Read the model definition and answer for the solid it produces. Units are mm, in the model's axes. A direction names the side the tool comes from. Coordinates: 2 decimals unless noted, no trailing zeros. Loops run counter-clockwise (first coordinate to the right, second up) from the corner with the lowest first, then second, coordinate; pieces in that order, holes last.
from build123d import *

# Parameters (mm, degrees)
F1_DEPTH = 7.5
F2_W     = 25
F2_H     = 2
F2_W_2   = 87.9392416629
F3_DEPTH = 127.501
F4_DEPTH = 7.5
F5_D     = 3
F5_DEPTH = 13.5
F5_TIP   = 0.9012909285
F7_R     = 2.6
F8_DEPTH = 15
F6_R     = 2.55
F9_DEPTH = 12.5


with BuildPart() as f1:
    # F0 (on Front) → F1 (new body, symmetric)
    with BuildSketch(Plane.XZ):
        with BuildLine():
            ThreePointArc((0, 127.5), (5.3033008589, 125.3033008589), (7.5, 120))
            ThreePointArc((7.5, 120), (5.3033008589, 114.6966991411), (0, 112.5))
            Line((0, 112.5), (108.7850481272, 112.5))
            Line((108.7850481272, 112.5), (108.7850481272, 127.5))
            Line((108.7850481272, 127.5), (0, 127.5))
        make_face()
        with BuildLine():
            Line((120, 127.5), (108.7850481272, 127.5))
            Line((108.7850481272, 127.5), (108.7850481272, 112.5))
            Line((108.7850481272, 112.5), (120, 112.5))
            ThreePointArc((120, 112.5), (127.5, 120), (120, 127.5))
        make_face()
        with BuildLine():
            ThreePointArc((0, 112.5), (5.3033008589, 114.6966991411), (7.5, 120))
            ThreePointArc((7.5, 120), (5.3033008589, 125.3033008589), (0, 127.5))
            ThreePointArc((0, 127.5), (-7.5, 120), (0, 112.5))
        make_face()
        with BuildLine():
            Line((162.6379891518, 127.5), (120, 127.5))
            ThreePointArc((120, 127.5), (127.5, 120), (120, 112.5))
            Line((120, 112.5), (124.3643918131, 112.5))
            ThreePointArc((124.3643918131, 112.5), (126.7854456219, 110.6232964421), (125.5716191931, 107.8107987637))
            Line((125.5716191931, 107.8107987637), (-3.6216821402, 36.5676037088))
            ThreePointArc((-3.6216821402, 36.5676037088), (3.813619275, 36.4580421202), (7.5, 30))
            ThreePointArc((7.5, 30), (6.4580421202, 26.186380725), (3.6216821402, 23.4323962912))
            Line((3.6216821402, 23.4323962912), (163.8452165318, 111.7871050513))
            ThreePointArc((163.8452165318, 111.7871050513), (164.7906698585, 112.7050998626), (165.1379891518, 113.9763062876))
            Line((165.1379891518, 113.9763062876), (165.1379891518, 125))
            ThreePointArc((165.1379891518, 125), (164.4057561047, 126.767766953), (162.6379891518, 127.5))
        make_face()
        with BuildLine():
            ThreePointArc((7.5, 30), (3.813619275, 36.4580421202), (-3.6216821402, 36.5676037088))
            ThreePointArc((-3.6216821402, 36.5676037088), (-6.5676037088, 26.3783178598), (3.6216821402, 23.4323962912))
            ThreePointArc((3.6216821402, 23.4323962912), (6.4580421202, 26.186380725), (7.5, 30))
        make_face()
    extrude(amount=F1_DEPTH, both=True)

    # F2 (on Top) → F3 (cut, through all)
    with BuildSketch(Plane.XY):
        with Locations((23.2615718412, 7.6191863865)):
            Rectangle(F2_W, F2_H)
        with Locations((-1.7384281588, 7.6191863865)):
            Rectangle(F2_W, F2_H)
        with Locations((261.2008135041, 7.6191863865)):
            Rectangle(F2_W, F2_H)
        with Locations((211.2008135041, 7.6191863865)):
            Rectangle(F2_W, F2_H)
        with Locations((48.2615718412, 7.6191863865)):
            Rectangle(F2_W, F2_H)
        with Locations((236.2008135041, 7.6191863865)):
            Rectangle(F2_W, F2_H)
        with Locations((186.2008135041, 7.6191863865)):
            Rectangle(F2_W, F2_H)
        with Locations((129.7311926726, 7.6191863865)):
            Rectangle(F2_W_2, F2_H)
        with Locations((73.2615718412, 7.6191863865)):
            Rectangle(F2_W, F2_H)
        with Locations((48.2615718412, 3.6191863865)):
            Rectangle(F2_W, F2_H)
        with Locations((73.2615718412, 3.6191863865)):
            Rectangle(F2_W, F2_H)
        with Locations((-1.7384281588, 3.6191863865)):
            Rectangle(F2_W, F2_H)
        with Locations((261.2008135041, 3.6191863865)):
            Rectangle(F2_W, F2_H)
        with Locations((23.2615718412, 3.6191863865)):
            Rectangle(F2_W, F2_H)
        with Locations((236.2008135041, 3.6191863865)):
            Rectangle(F2_W, F2_H)
        with Locations((129.7311926726, 3.6191863865)):
            Rectangle(F2_W_2, F2_H)
        with Locations((186.2008135041, 3.6191863865)):
            Rectangle(F2_W, F2_H)
        with Locations((211.2008135041, 3.6191863865)):
            Rectangle(F2_W, F2_H)
        with Locations((261.2008135041, -0.3808136135)):
            Rectangle(F2_W, F2_H)
        with Locations((129.7311926726, -0.3808136135)):
            Rectangle(F2_W_2, F2_H)
        with Locations((48.2615718412, -0.3808136135)):
            Rectangle(F2_W, F2_H)
        with Locations((73.2615718412, -0.3808136135)):
            Rectangle(F2_W, F2_H)
        with Locations((-1.7384281588, -0.3808136135)):
            Rectangle(F2_W, F2_H)
        with Locations((23.2615718412, -0.3808136135)):
            Rectangle(F2_W, F2_H)
        with Locations((236.2008135041, -0.3808136135)):
            Rectangle(F2_W, F2_H)
        with Locations((186.2008135041, -0.3808136135)):
            Rectangle(F2_W, F2_H)
        with Locations((211.2008135041, -0.3808136135)):
            Rectangle(F2_W, F2_H)
        with Locations((236.2008135041, -4.3808136135)):
            Rectangle(F2_W, F2_H)
        with Locations((261.2008135041, -4.3808136135)):
            Rectangle(F2_W, F2_H)
        with Locations((48.2615718412, -4.3808136135)):
            Rectangle(F2_W, F2_H)
        with Locations((73.2615718412, -4.3808136135)):
            Rectangle(F2_W, F2_H)
        with Locations((129.7311926726, -4.3808136135)):
            Rectangle(F2_W_2, F2_H)
        with Locations((186.2008135041, -4.3808136135)):
            Rectangle(F2_W, F2_H)
        with Locations((211.2008135041, -4.3808136135)):
            Rectangle(F2_W, F2_H)
        with Locations((23.2615718412, -4.3808136135)):
            Rectangle(F2_W, F2_H)
        with Locations((-1.7384281588, -4.3808136135)):
            Rectangle(F2_W, F2_H)
    extrude(amount=F3_DEPTH, mode=Mode.SUBTRACT)

    # F0 (on Front) → F4 (join, symmetric)
    with BuildSketch(Plane.XZ):
        with BuildLine():
            ThreePointArc((0, 112.5), (5.3033008589, 114.6966991411), (7.5, 120))
            ThreePointArc((7.5, 120), (5.3033008589, 125.3033008589), (0, 127.5))
            ThreePointArc((0, 127.5), (-7.5, 120), (0, 112.5))
        make_face()
        with BuildLine():
            Line((120, 127.5), (108.7850481272, 127.5))
            Line((108.7850481272, 127.5), (108.7850481272, 112.5))
            Line((108.7850481272, 112.5), (120, 112.5))
            ThreePointArc((120, 112.5), (127.5, 120), (120, 127.5))
        make_face()
        with BuildLine():
            ThreePointArc((7.5, 30), (3.813619275, 36.4580421202), (-3.6216821402, 36.5676037088))
            ThreePointArc((-3.6216821402, 36.5676037088), (-6.5676037088, 26.3783178598), (3.6216821402, 23.4323962912))
            ThreePointArc((3.6216821402, 23.4323962912), (6.4580421202, 26.186380725), (7.5, 30))
        make_face()
    extrude(amount=F4_DEPTH, both=True)

    # F5 (one way)
    with BuildSketch(Plane.XZ):
        with Locations((0, 120), (0, 30)):
            Circle(F5_D / 2)
    extrude(amount=-F5_DEPTH, mode=Mode.SUBTRACT)
    with Locations(Plane.XZ):
        with Locations((0, 120), (0, 30)):
            with Locations((0, 0, -(F5_DEPTH + F5_TIP / 2))):  # 118° drill point
                Cone(0, F5_D / 2, F5_TIP, mode=Mode.SUBTRACT)

    # F7 (on face) → F8 (cut, through all)
    with BuildSketch(Plane.XY.offset(127.5)):
        with Locations((114.0677630901, 0)):
            Circle(F7_R)
    extrude(amount=-F8_DEPTH, mode=Mode.SUBTRACT)

    # F6 (on Front) → F9 (cut, symmetric)
    with BuildSketch(Plane.XZ):
        with Locations((0, 120)):
            Circle(F6_R)
        with Locations((0, 30)):
            Circle(F6_R)
    extrude(amount=F9_DEPTH, both=True, mode=Mode.SUBTRACT)


solid = f1.part
Q1. A cutting plane is placed at C-C (z = 60.5). Give the vertices of the cut face in (x, y).
Findings below:
outline: (39.78, -7.5) - (70.84, -7.5) - (70.84, -5.38) - (39.78, -5.38) - close; (39.78, -3.38) - (70.84, -3.38) - (70.84, -1.38) - (39.78, -1.38) - close; (39.78, 0.62) - (70.84, 0.62) - (70.84, 2.62) - (39.78, 2.62) - close; (39.78, 4.62) - (70.84, 4.62) - (70.84, 6.62) - (39.78, 6.62) - close
Q2. Which of the six approach directions +Z, -Z, +X, -X, +Y, -Y give full straight-line access (tool end or side, diameter ignored) to faces 1 (the face through (111.47, 0.11, 120.1)), 2 (the face through (0, 7.5, 117)), 3 (the face through (61.9, 5.6, 72.7)), 4 (the face through (127.5, -4.37, 119.84))?
Findings below:
face 1: +Z
face 2: +Z, -Z, +X, -X, +Y
face 3: -X, +Y, -Y
face 4: +X
Q3. Straight lines are drawn through the part: probe 1 along Y at (x, z) = (10.5, 36.5); probe 2 along X at (y, z) = (-5, 120); probe 3 along Z at (x, y) = (0, -5). For each, find the intervals that lie inside material, in ascending order.
Findings below:
probe 1: y = -7.5 to -5.38, -3.38 to -1.38, 0.62 to 2.62, 4.62 to 6.62
probe 2: x = -7.5 to -2.55, 2.55 to 7.5, 108.79 to 127.5
probe 3: z = 22.5 to 27.45, 32.55 to 37.5, 112.5 to 117.45, 122.55 to 127.5
Q4. Determine the mould class of faces 5 (the face through (61.9, -6.5, 72.7)), 6 (the face through (3, 7.5, 30)), 7 (the face through (127.5, -0.37, 119.84)) for opening direction Z: +Z half, -Z half, draft (parallel to the pull), parting line (faces both ways), or undercut.
Findings below:
face 5: undercut
face 6: draft
face 7: parting line
Q5. Flat-ended cylindrical pins translate along their axes: pin 1 Ø1 at (x, y) = (113, 6) entering from -Z; pin 2 Ø1.6 at (x, y) = (112, 4) entering from -Z; pin 3 Ø1 at (y, z) = (2.5, 61.5) entering from +X; pin 4 Ø3 at (x, z) = (0, 120) entering from -Y. Find the tip coordinate at first contact, or state that the pin passes through.
Findings below:
pin 1: stops at z = 83.47
pin 2: stops at z = 82.92
pin 3: stops at x = 73.56
pin 4: passes through
Q6. A cutting plane is placed at A-A (z = 120). Count the separate pieces of the cut face and the enclosed holes in it, then the cut area to 3 significant figures.
Findings below:
separate pieces: 2
enclosed holes: 4
area: 1,540 mm2
